Verification items for this drawing (mm, ordinates from the low corner). A direction names the side the tool comes from. Coordinates: 2 decimals unless noted, no trailing zeros. Loops run counter-clockwise (first coordinate to the right, second up) from the corner with the lowest first, then second, coordinate; pieces in that order, holes last. Notation, with made-up numbers: (1, 26.5) -> (11, 26.5) arc R24 ccw to (11, 62.5) -> close; hole circle Ø3 at (-20.5, 22.5). An arc over 180 degrees is marked (long way). Write item = value, one per line.
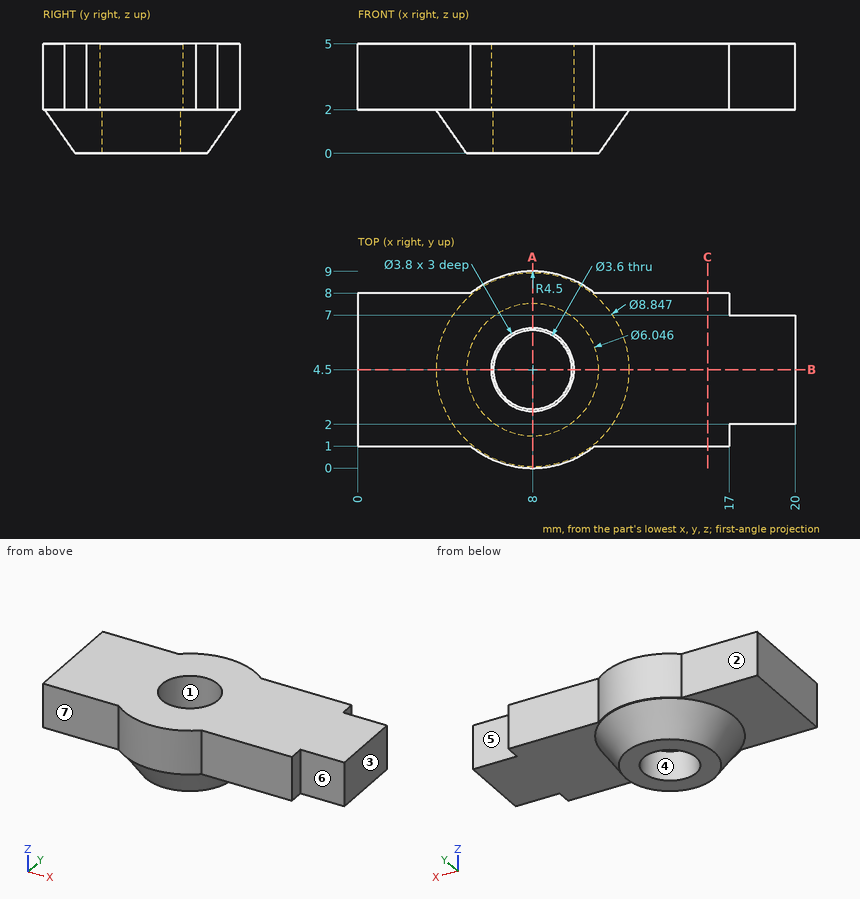
1) Sectioned sample at C-C, the plane x = 16. Record the cut outline in (y, z).
Ans:
outline = (1, 2) -> (8, 2) -> (8, 5) -> (1, 5) -> close
2) Sectioned sample at A-A, the plane x = 8. Record the cut outline in (y, z), plus the area to 3 significant figures.
Ans:
outline = (0, 2) -> (0.08, 2) -> (1.48, 0) -> (2.7, 0) -> (2.7, 2) -> (2.6, 2) -> (2.6, 5) -> (0, 5) -> close; (6.3, 0) -> (7.52, 0) -> (8.92, 2) -> (9, 2) -> (9, 5) -> (6.4, 5) -> (6.4, 2) -> (6.3, 2) -> close
area = 23.3 mm2
3) Release check for a two-part mould opening along X. For the marked faces 1, 2, 3 and 4 record: pulls with the +X half, pulls with the -X half, needs draft (parallel to the pull), parting line crosses it, or undercut.
Ans:
face_1 = undercut
face_2 = needs draft
face_3 = pulls with the +X half
face_4 = undercut
4) Material ranges on line 1 (Y direction, x = 8, z = 3.4); line 2 (X direction, y = 4.5, z = 3.45); line 3 (Z direction, x = 3.25, y = 3.5), recorded low to high.
Ans:
line_1 = 0 to 2.6, 6.4 to 9
line_2 = 0 to 6.1, 9.9 to 20
line_3 = 2 to 5
5) Tool access check on the marked faces 5, 6 and 7. Record the directions out of +Z, -Z, +X, -X, +Y, -Y that give a thin tool (end or side, any length) a straight path to the whole face; none if there is none.
Ans:
face_5 = +Z, -Z, +X, +Y
face_6 = +Z, -Z, +X, -Y
face_7 = +Z, -Z, -X, -Y
6) Depth check by flat-ended pin: pin 1 Ø1.5 at (x, z) = (1.5, 4) entering from +Y; pin 2 Ø0.9 at (x, z) = (18, 3) entering from +Y; pin 3 Ø4.5 at (x, y) = (14.5, 6.5) entering from -Z. Enter the tip coordinate at first touch or a pass-through.
Ans:
pin_1 = 8
pin_2 = 7
pin_3 = 2
7) Sectioned sample at B-B, the plane y = 4.5. Record the cut outline in (x, z).
Ans:
outline = (0, 2) -> (3.58, 2) -> (4.98, 0) -> (6.2, 0) -> (6.2, 2) -> (6.1, 2) -> (6.1, 5) -> (0, 5) -> close; (9.8, 0) -> (11.02, 0) -> (12.42, 2) -> (20, 2) -> (20, 5) -> (9.9, 5) -> (9.9, 2) -> (9.8, 2) -> close
